```python
from build123d import *

# Parameters (mm, degrees)
F0_W     = 111.125
F0_H     = 25.4
F1_DEPTH = 4.7498
F2_R     = 12.69999
F3_R     = 3.5
F3_R_2   = 3.5052
F4_DEPTH = 25.4


# Not quite as in the source:
# - a fillet or chamfer is up to 0.001 mm smaller than in the source, because OpenCascade refuses the exact size


with BuildPart() as f1:
    # F0 (on Top) → F1 (new body)
    with BuildSketch(Plane.XY):
        Rectangle(F0_W, F0_H)
    extrude(amount=F1_DEPTH)

    # F2 (radius 12.7 in the source; OpenCascade refuses exactly that, so slightly less here)
    f2_edges = [f1.edges().sort_by_distance(p)[0] for p in [
        (-55.5625, -12.7, 2.3749),
        (-55.5625, 12.7, 2.3749),
        (55.5625, -12.7, 2.3749),
        (55.5625, 12.7, 2.3749),
    ]]
    fillet(f2_edges, radius=F2_R)

    # F3 (on face) → F4 (cut)
    with BuildSketch(Plane.XY.offset(4.7498)):
        with Locations((-42.8625, 0)):
            Circle(F3_R)
        with Locations((42.8625, 0)):
            Circle(F3_R_2)
    extrude(amount=-F4_DEPTH, mode=Mode.SUBTRACT)


solid = f1.part
```
Build history of the part. All positions in model axes, mm. Give positions to 0.01 mm unless a question says otherwise; leave off trailing zeros. Loops run counter-clockwise (first coordinate to the right, second up) from the corner with the lowest first, then second, coordinate; pieces in that order, holes last. Notation, with made-up numbers: (4, 68.5) -> (29, 68.5) arc R8 ccw to (29, 79.5) -> close; hole circle Ø11 at (82, -36.5). An arc over 180 degrees is marked (long way). One line per question, with ' | ' between items. Start each with the question number.
1) Cut at B-B (z = 2.95). Count the separate pieces of the cut face and the enclosed holes in it, plus the area to 3 significant figures.
2) Cut at D-D (y = 8.5). Give the cut face in (x, z), plus the area to 3 significant figures.
3) Cut at A-A (y = 1.5). Give the cut face in (x, z).
4) Pin check, flat tips, straight feed: pin 1 (1 mm diameter, centred on y = 1, z = 1, fed in from +X); pin 2 (6.5 mm diameter, centred on x = -42.86, y = 0, fed in from -Z). Stop position of each tip, or through.
5) Two-plate mould, pull along X, no slides. Class faces 1 (the cylindrical face through (-39.524, 1.051, 2.408)), 2 (the cylindrical face through (46.206, 1.053, 2.408)), 3 (the flat face through (-1, -12.7, 2)), 4 (the cylindrical face through (-51.94, -8.88, 2.41)): released by +X, released by -X, zero draft, split by the parting line, or undercut.
6) Cut at C-C (x = 44.5). Give the cut face in (y, z), plus the area to 3 significant figures.
7) Probe L1, parallel to X at y = 3, z = 0.6; L2, parallel to Y at x = -46, z = 1.45; L3, parallel to X at y = 4.5, z = 1.2. List the from-to ranges inside material, lowest first.
Return value:
1) separate pieces: 1 | enclosed holes: 2 | area: 2,610 mm^2
2) outline: (-52.3, 0) -> (52.3, 0) -> (52.3, 4.75) -> (-52.3, 4.75) -> close | area: 497 mm^2
3) outline: (-55.47, 0) -> (-46.02, 0) -> (-46.02, 4.75) -> (-55.47, 4.75) -> close; (-39.7, 0) -> (39.69, 0) -> (39.69, 4.75) -> (-39.7, 4.75) -> close; (46.03, 0) -> (55.47, 0) -> (55.47, 4.75) -> (46.03, 4.75) -> close
4) pin 1: x = 55.55 | pin 2: through
5) face 1: undercut | face 2: undercut | face 3: zero draft | face 4: released by -X
6) outline: (-12.59, 0) -> (-3.1, 0) -> (-3.1, 4.75) -> (-12.59, 4.75) -> close; (3.1, 0) -> (12.59, 0) -> (12.59, 4.75) -> (3.1, 4.75) -> close | area: 90.2 mm^2
7) L1: -55.2 to -44.67, -41.06 to 41.05, 44.68 to 55.2 | L2: -12.31 to -1.55, 1.55 to 12.31 | L3: -54.74 to 54.74
